Autodesk Inventor part; units mm, degrees
ref_plane "YZ Plane" through (0, 0, 0) normal (1, 0, 0) x (0, 1, 0)
ref_plane "XZ Plane" through (0, 0, 0) normal (0, 1, 0) x (-1, 0, 0)
ref_plane "XY Plane" through (0, 0, 0) normal (0, 0, 1) x (1, 0, 0)
sketch "スケッチ1" plane through (0, 0, 0) normal (0, 0, 1) x (1, 0, 0)
  line L0 (-34.7, 15.2) -> (34.7, 15.2)
  line L1 (34.7, 15.2) -> (34.7, -15.2)
  line L2 (34.7, -15.2) -> (-34.7, -15.2)
  line L3 (-34.7, -15.2) -> (-34.7, 15.2)
  line L4 (-30.85, 11.35) -> (30.85, 11.35) construction
  line L5 (30.85, 11.35) -> (30.85, -11.35) construction
  line L6 (30.85, -11.35) -> (-30.85, -11.35) construction
  line L7 (-30.85, -11.35) -> (-30.85, 11.35) construction
  circle A0 centre (-30.85, 11.35) radius 1.25
  circle A1 centre (-30.85, -11.35) radius 1.25
  circle A2 centre (30.85, -11.35) radius 1.25
  circle A3 centre (30.85, 11.35) radius 1.25
  line L8 (36.7, 17.2) -> (-36.7, 17.2)
  line L9 (-36.7, 17.2) -> (-36.7, -17.2)
  line L10 (-36.7, -17.2) -> (36.7, -17.2)
  line L11 (36.7, -17.2) -> (36.7, 17.2)
  point P0 (0, 0)
  point P1 (0, 15.2)
  point P2 (-34.7, 0)
  point P3 (0, 11.35)
  point P4 (-30.85, 0)
  dimension "d0" = 30.4
  dimension "d1" = 69.4
  dimension "d2" = 61.7
  dimension "d3" = 22.7
  dimension "d4" = 2.5
  dimension "d5" = 2
extrude "押し出し1" add sketch "スケッチ1" along normal blind 1.6 contours L11 L10 L9 L8
extrude "押し出し2" add sketch "スケッチ1" against normal blind 2.4 contours L0 L1 L2 L3 | L11 L10 L9 L8
sketch "スケッチ2" plane through (0, 0, 0) normal (0, 0, 1) x (1, 0, 0)
  circle A0 centre (-30.85, -11.35) radius 1.25 construction
  circle A1 centre (-30.85, 11.35) radius 1.25 construction
  circle A2 centre (30.85, -11.35) radius 1.25 construction
  circle A3 centre (30.85, 11.35) radius 1.25 construction
  line L0 (-34.7, -15.2) -> (-34.7, 15.2)
  line L1 (34.7, -15.2) -> (-34.7, -15.2)
  line L2 (-34.7, 15.2) -> (34.7, 15.2)
  line L3 (34.7, 15.2) -> (34.7, -15.2)
  line L4 (-27.85, -15.2) -> (-27.85, -11.35)
  arc A4 (-27.85, -11.35) -> (-30.85, -8.35) centre (-30.85, -11.35) ccw
  line L5 (-30.85, -8.35) -> (-34.7, -8.35)
  line L6 (-34.7, 8.35) -> (-30.85, 8.35)
  arc A5 (-30.85, 8.35) -> (-27.85, 11.35) centre (-30.85, 11.35) ccw
  line L7 (-27.85, 11.35) -> (-27.85, 15.2)
  line L8 (27.85, -15.2) -> (27.85, -11.35)
  arc A6 (30.85, -8.35) -> (27.85, -11.35) centre (30.85, -11.35) ccw
  line L9 (30.85, -8.35) -> (34.7, -8.35)
  line L10 (34.7, 8.35) -> (30.85, 8.35)
  arc A7 (27.85, 11.35) -> (30.85, 8.35) centre (30.85, 11.35) ccw
  line L11 (27.85, 11.35) -> (27.85, 15.2)
  point P0 (0, 0)
  dimension "d10" = 3
extrude "押し出し3" cut sketch "スケッチ2" against normal blind 1.2 contours L0 L6 A5 L7 L2 L11 A7 L10 L3 L9 A6 L8 L1 L4 A4 L5
sketch "スケッチ3" plane through (0, 0, -2.4) normal (0, 0, -1) x (-1, 0, 0)
  circle A0 centre (-30.85, 11.35) radius 1.25 construction
  circle A1 centre (-30.85, -11.35) radius 1.25 construction
  line L0 (-30.85, 23.2) -> (-30.85, -23.2) construction
  line L1 (-25, 23.2) -> (-25, -23.2)
  line L2 (-36.7, -23.2) -> (-36.7, 23.2)
  arc A2 (-25, 23.2) -> (-36.7, 23.2) centre (-30.85, 23.2) ccw
  arc A3 (-36.7, -23.2) -> (-25, -23.2) centre (-30.85, -23.2) ccw
  line L3 (36.7, 17.2) -> (-36.7, 17.2)
  line L4 (-36.7, -17.2) -> (36.7, -17.2)
  circle A4 centre (-30.85, 23.2) radius 2.25
  circle A5 centre (-30.85, -23.2) radius 2.25
  line L5 (-30.85, 29.05) -> (-26.85, 29.05)
  arc A6 (-22.7134, 27.3366) -> (-26.85, 29.05) centre (-26.85, 23.2) ccw
  line L6 (-22.7134, 27.3366) -> (-12.5769, 17.2)
  line L7 (-36.7, 17.2) -> (36.7, 17.2)
  line L8 (-30.85, -29.05) -> (-26.85, -29.05)
  arc A7 (-26.85, -29.05) -> (-22.7134, -27.3366) centre (-26.85, -23.2) ccw
  line L9 (-22.7134, -27.3366) -> (-12.5769, -17.2)
  point P0 (0, 0)
  point P1 (-30.85, 0)
  dimension "d14" = 6
  dimension "d15" = 6
  dimension "d16" = 46.4
  dimension "d17" = 4.5
  dimension "d18" = 45
  dimension "d19" = 4
extrude "押し出し4" add sketch "スケッチ3" against normal up to surface (4 mm away) contours A2 L5 A6 L6 L3 L1 | L1 L3 L2 A2 | L4 L9 A7 L8 A3 L1 | L1 A3 L2 L4
fillet "フィレット2" radius 3 2 edges at (12.5769, -17.2, -0.4) (12.5769, 17.2, -0.4)
fillet "フィレット1" radius 2 2 edges at (-36.7, 17.2, -0.4) (-36.7, -17.2, -0.4)
equation "\"d15\" = d14"
properties part number "power_sync_module_case"
Geometry check sheet. Reference: the model listing, model coordinates, mm. A direction names the side the tool comes from. Round coordinates to 2 decimals unless told otherwise and drop trailing zeros. Loops run counter-clockwise (first coordinate to the right, second up) from the corner with the lowest first, then second, coordinate; pieces in that order, holes last. Notation, with made-up numbers: (82, 28.25) -> (131, 28.25) arc R17 ccw to (131, 54.25) -> close; hole circle Ø2 at (-29, 61). An arc over 180 degrees is marked (long way). Answer as a JSON object with one key per item and string values. Group by question number.
Item 1: Thickness scan on line 1 along Y through (x, z) = (30.85, 0.35); line 2 along Y through (x, z) = (30.85, -0.25); line 3 along Y through (x, z) = (30.85, -1.5). Record the ranges inside material, lowest first.
Item 2: Release check for a two-part mould opening along Y. For faces 1 (the face through (13, -17, 1.6)), 2 (the face through (-11, 17.2, 0)), 3 (the face through (32, -12.5, 0)), 4 (the face through (18.149, -22.772, -0.428)) record: pulls with the +Y half, pulls with the -Y half, needs draft (parallel to the pull), parting line crosses it, or undercut.
Item 3: Cross-section at A-A, the plane y = 0. Record the cut outline in (x, z), plus the area to 3 significant figures.
Item 4: Cross-section at B-B, the plane x = -9. Record the cut outline in (y, z).
Item 5: Set-up check for faces 5 (the face through (-12, -17.2, 0)), 6 (the face through (-31, 13, 0)), 7 (the face through (28.77, 22.34, -0.43)): record each of +Z, -Z, +X, -X, +Y, -Y from which the full face is reachable in a straight line by a thin tool's end or side.
Item 6: Depth check by flat-ended pin: pin 1 Ø0.6 at (x, z) = (32, -1) entering from +Y; pin 2 Ø1.5 at (x, z) = (0, -0.5) entering from -Y; pin 3 Ø1.3 at (x, z) = (-33, -0.5) entering from +Y; pin 4 Ø2 at (x, y) = (-30.85, 11.35) entering from -Z. Enter the tip coordinate at first touch or a pass-through.
Determined:
{
 "1": {"line 1": "y = -29.05 to -25.45, -20.95 to -15.2, 15.2 to 20.95, 25.45 to 29.05", "line 2": "y = -29.05 to -25.45, -20.95 to -12.6, -10.1 to -8.35, 8.35 to 10.1, 12.6 to 20.95, 25.45 to 29.05", "line 3": "y = -29.05 to -25.45, -20.95 to -12.6, -10.1 to 10.1, 12.6 to 20.95, 25.45 to 29.05"},
 "2": {"face 1": "needs draft", "face 2": "pulls with the +Y half", "face 3": "undercut", "face 4": "pulls with the -Y half"},
 "3": {"outline": "(-36.7, -2.4) -> (36.7, -2.4) -> (36.7, 1.6) -> (34.7, 1.6) -> (34.7, -1.2) -> (-34.7, -1.2) -> (-34.7, 1.6) -> (-36.7, 1.6) -> close", "area": "99.3 mm²"},
 "4": {"outline": "(-17.2, -2.4) -> (17.2, -2.4) -> (17.2, 1.6) -> (15.2, 1.6) -> (15.2, -1.2) -> (-15.2, -1.2) -> (-15.2, 1.6) -> (-17.2, 1.6) -> close"},
 "5": {"face 5": "+Z, -Z, -X, -Y", "face 6": "+Z", "face 7": "+Z, -Z"},
 "6": {"pin 1": "stops at y = 28.99", "pin 2": "stops at y = -17.2", "pin 3": "stops at y = 17.2", "pin 4": "passes through"}
}
